For this review, take the finished solid that the model builds, in its own axes (mm). Face numbers are marked on the shaded views. A direction names the side the tool comes from. Give positions to 0.01 mm unless a question says otherwise; leave off trailing zeros. Order: outer loops, then holes, each group sorted by start corner. A loop starts at its lowest first (then second) coordinate and runs counter-clockwise, first axis right, second up. Notation, with made-up numbers: M -11.5,69 L 47.5,69 A26 ccw 47.5,90 Z; hole C 13,85.5 d7. An arc over 180 degrees is marked long. Use CSV: the item, a comma, the result in double quotes. Start each with the question number.
(1) Consider section D-D (z = 1). Write out the cut boundary in (x, y), and give its area (3 significant figures).
(2) Tool access review of the marked faces 1 and 2: name each direction out of +Z, -Z, +X, -X, +Y, -Y from which nothing blocks a thin tool from reaching the whole face with its end or side.
(3) Wall thickness on L1, parallel to X at y = 6, z = 22.5; L2, parallel to Z at x = 14.5, y = 5.5: over which ranges is each line inside the solid? List them lowest first. Write a range as from..to.
(4) Clearance check with flat-ended pins moving along their axes: P1, Ø18.5, axis at y = 40.5, z = -8, coming from the -X side; P2, Ø5, axis at x = 13.5, y = 33.5, coming from the +Z side. State where each tip first meets the part, or that it passes through.
(5) Consider section B-B (y = 19.5). Write out the cut boundary in (x, z), and give its area (3 significant figures).
(6) Consider section A-A (x = 3). Write out the cut boundary in (y, z).
(7) Consider section C-C (x = 23). Write out the cut boundary in (y, z), and give its area (3 significant figures).
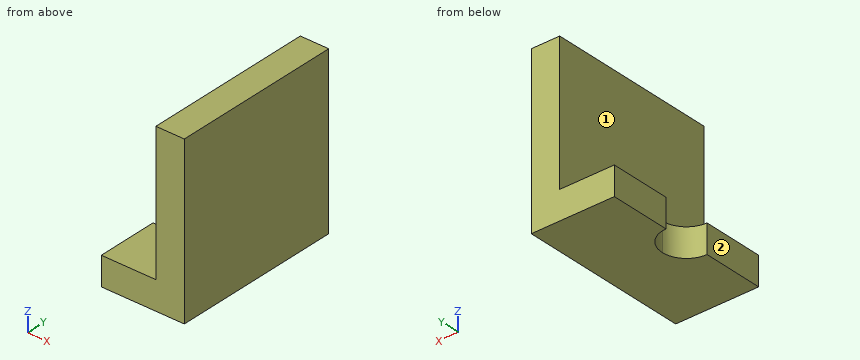
```python
from build123d import *

# Parameters (mm, degrees)
F1_DEPTH = 76.2
F3_DEPTH = 39.624


with BuildPart() as f1:
    # F0 (on Front) → F1 (new body)
    with BuildSketch(Plane.XZ):
        Polygon((0, -30.248137), (0, -42.948137), (37.062691, -42.948137), (37.062691, 31.328041), (24.362691, 31.328041), (24.362691, -30.248137), align=None)
    extrude(amount=-F1_DEPTH)

    # F2 (on face) → F3 (cut)
    with BuildSketch(Plane.XY.offset(-30.248137)):
        with BuildLine():
            ThreePointArc((0, 27.292805), (7.641841, 30.458159), (10.807195, 38.1))
            ThreePointArc((10.807195, 38.1), (7.641841, 45.741841), (0, 48.907195))
            Line((0, 48.907195), (0, 27.292805))
        make_face()
    extrude(amount=-F3_DEPTH, mode=Mode.SUBTRACT)


solid = f1.part
```
Check result:
1,outline,"M 24.36,0 L 37.06,0 L 37.06,76.2 L 24.36,76.2 Z"
1,area,"968 mm^2"
2,face 1,"+Z, -X, +Y, -Y"
2,face 2,"+Z, -Z, -X, +Y, -Y"
3,L1,"x = 24.36..37.06"
3,L2,"z = -42.95..-30.25"
4,P1,"stops at x = 24.36"
4,P2,"stops at z = -30.25"
5,outline,"M 0,-42.95 L 37.06,-42.95 L 37.06,31.33 L 24.36,31.33 L 24.36,-30.25 L 0,-30.25 Z"
5,area,"1,250 mm^2"
6,outline,"M 0,-42.95 L 27.72,-42.95 L 27.72,-30.25 L 0,-30.25 Z; M 48.48,-42.95 L 76.2,-42.95 L 76.2,-30.25 L 48.48,-30.25 Z"
7,outline,"M 0,-42.95 L 76.2,-42.95 L 76.2,-30.25 L 0,-30.25 Z"
7,area,"968 mm^2"
